Source: CAD feature listing. Evaluate the final solid. Frame: model axes, mm. Face numbers are marked on the shaded views. A direction names the side the tool comes from. Coordinates: 2 decimals unless noted, no trailing zeros. Write each loop counter-clockwise with the first axis right and the second up, starting at its lowest first coordinate (ties: lowest second). Pieces come first, ordered by that corner, then holes. Notation, with made-up numbers: (23.25, 73.25) -> (79.25, 73.25) arc R37 cw to (79.25, 112.25) -> close; hole circle Ø8 at (54.5, -15). An arc over 180 degrees is marked (long way). One line per item, written item: value. Start each with the question number.
1. Section query B-B, the plane z = 15.5. Output: boundary loops of the cut face in (x, y), and give its area (3 significant figures).
2. Line query: line 1 (Y direction, x = 0, z = 6); line 2 (X direction, y = 0, z = 15); line 3 (X direction, y = 0, z = 28.25). Output: solid intervals per line, ascending.
3. Access query for the marked faces 1, 2, 3 and 4. Directions: +Z, -Z, +X, -X, +Y, -Y. A direction counts if a zero-diameter tool reaches every point of the face in a straight line with its end or side. Return the directions, or none.
4. Section query C-C, the plane x = 0. State how many separate pieces and enclosed holes the cut face has, and give its area (3 significant figures).
5. Section query D-D, the plane y = -28. Output: boundary loops of the cut face in (x, z).
6. First-contact query: P1, Ø12, axis at x = 17.5, z = 15, coming from the +Y side; P2, Ø2, axis at y = -2.5, z = 9.5, coming from the -X side; P3, Ø4, axis at x = -13, z = 5.5, coming from the -Y side. Flat tips, straight axial feed; report the tip coordinate or a pass-through.
Autodesk Inventor part; units mm, degrees
ref_plane "Arbeitsebene1" through (35, 0, 10) normal (1, 0, 0) x (0, 1, 0)
ref_plane "XZ Plane" through (0, 0, 0) normal (0, 1, 0) x (-1, 0, 0)
ref_plane "XY Plane" through (0, 0, 0) normal (0, 0, 1) x (1, 0, 0)
sketch "Skizze1" plane through (0, 0, 0) normal (0, 1, 0) x (-1, 0, 0)
  line L0 (17, 30.75) -> (17, 26.75)
  line L1 (17, 26.75) -> (20, 26.75)
  line L2 (20, 26.75) -> (20, 6.75)
  line L3 (23, 0) -> (35, 0)
  line L4 (35, 0) -> (35, 20)
  line L5 (35, 20) -> (25, 20)
  line L6 (25, 20) -> (25, 30.75)
  line L7 (17, 30.75) -> (25, 30.75)
  line L8 (0, 0) -> (0, 48.4152)
  line L9 (20, 6.75) -> (23, 6.75)
  line L10 (23, 6.75) -> (23, 4.75)
  line L11 (23, 4.75) -> (25, 4.75)
  line L12 (25, 4.75) -> (25, 3)
  line L13 (25, 3) -> (23, 3)
  line L14 (23, 3) -> (23, 0)
  point P0 (17, 4)
  dimension "d1" = 40
  dimension "d3" = 20
  dimension "d4" = 70
  dimension "d5" = 50
  dimension "d7" = 4
  dimension "d10" = 2
  dimension "d11" = 1.75
  dimension "d12" = 3
  dimension "d13" = 3
  dimension "d14" = 2
  dimension "d15" = 34
  dimension "d16" = 20
revolve "Umdrehung1" add sketch "Skizze1" angle 360 about axis through (0, 0, 0) along (0, 0, 1)
ref_plane "Arbeitsebene1" through (35, 0, 10) normal (1, 0, 0) x (0, 1, 0)
sketch "Skizze5" plane through (35, 0, 10) normal (1, 0, 0) x (0, 1, 0)
  line L0 (-36.029, 7.6022) -> (-33.5, 7.6022)
  line L1 (-33.5, 7.6022) -> (-33.5, -10.6796)
  line L2 (-33.5, -10.6796) -> (-36.029, -10.6796)
  line L3 (-36.029, -10.6796) -> (-36.029, 7.6022)
  line L4 (0, 27.0359) -> (0, -16.9655)
  point P0 (0, -10)
  dimension "d37" = 33.5
extrude "Extrusion3" cut sketch "Skizze5" against normal through all
sketch "Skizze6" plane through (-10.1366, -33.5, 0) normal (0, -1, 0) x (1, 0, 0)
  line L0 (20.2731, 0) -> (0, 0)
  point P0 (10.1366, 0)
  point P1 (10.1366, 12)
  dimension "d47" = 12
hole "Bohrung2" at (0, -33.5, 12) direction (0, 1, 0) diameter 5 end up to surface
thread "Gewinde1"
chamfer "Fase2" distance 1 angle 45 1 edges at (25, 0, 30.75)
properties part number "KON_Nietmaschine_Deckel" material "Stahl"
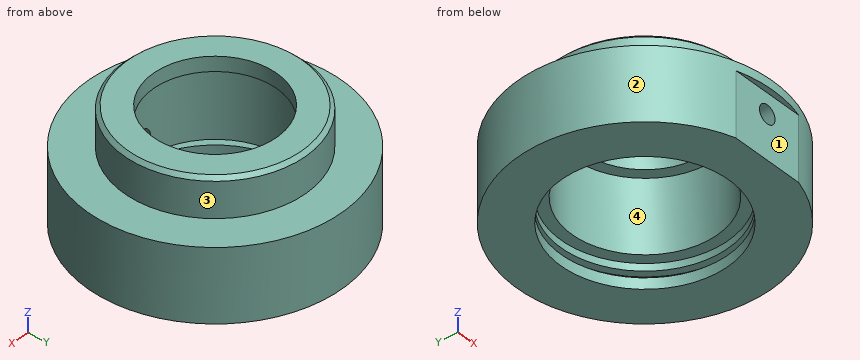
Computed values:
1. outline: (-10.14, -33.5) -> (10.14, -33.5) arc R35 ccw (long way) to start; hole circle Ø40 at (0, 0)
1. area: 2,570 mm²
2. line 1: y = -33.5 to -23, 23 to 35
2. line 2: x = -35 to -20, 20 to 35
2. line 3: x = -25 to -17, 17 to 25
3. face 1: -Z, +X, -X, -Y
3. face 2: +Z, -Z
3. face 3: +Z
3. face 4: -Z
4. separate pieces: 3
4. enclosed holes: 0
4. area: 589 mm²
5. outline: (-21, 0) -> (21, 0) -> (21, 20) -> (-21, 20) -> close; hole circle Ø5 at (0, 12)
6. P1: stops at y = 33.06
6. P2: stops at x = -34.97
6. P3: stops at y = -33.23
